The listing builds one solid part. Answer for the finished solid, in the listing's coordinates (mm). Face numbers are marked on the shaded views. Give positions to 0.01 mm unless a question says otherwise; leave off trailing zeros. Order: outer loops, then holes, each group sorted by start corner. A loop starts at its lowest first (then second) coordinate and runs counter-clockwise, first axis right, second up. Notation, with made-up numbers: (-8.75, -35) - (13.25, -35) arc R30 ccw to (13.25, -8) - close; hole circle Ø9 at (15, 28). An arc over 180 degrees is marked (long way). Answer in a Markdown table with one row per item. Add a question column.
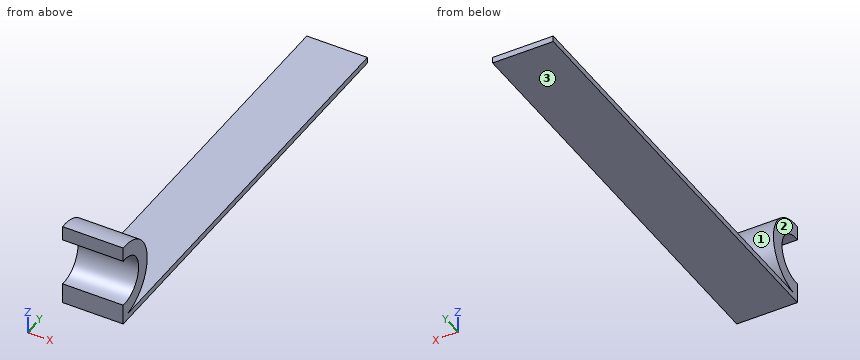
```python
from build123d import *

# Parameters (mm, degrees)
F0_W     = 25.4
F0_H     = 177.8
F1_DEPTH = 2.54
F4_DEPTH = 25.4


with BuildPart() as f1:
    # F0 (on Top) → F1 (new body)
    with BuildSketch(Plane.XY):
        with Locations((-51.181969, 33.563137)):
            Rectangle(F0_W, F0_H)
    extrude(amount=F1_DEPTH)

    # F3 (on face) → F4 (join)
    with BuildSketch(Plane.YZ.offset(-63.881969)):
        with BuildLine():
            Line((-55.336863, 8.636), (-55.336863, 2.54))
            ThreePointArc((-55.336863, 2.54), (-37.867352, 18.739499), (-55.336863, 34.938998))
            Line((-55.336863, 34.938998), (-55.336863, 28.842998))
            ThreePointArc((-55.336863, 28.842998), (-44.106861, 18.739499), (-55.336863, 8.636))
        make_face()
    extrude(amount=F4_DEPTH)


solid = f1.part
```
(1) The mould has two halves that part along Z. Classify the marked faces 1, 2 and 3: +Z half, -Z half, draft (parallel to the pull), parting line (faces both ways), or undercut.
(2) Each of these flat-tipped pins is pushed along its axis until it touches: P1, Ø6, axis at x = -52, z = 13.5, coming from the +Y side; P2, Ø3, axis at x = -52, y = 74, coming from the +Z side; P3, Ø1.5, axis at x = -43.5, z = 5, coming from the +Y side. Where does it stop, or does it pass through?
(3) Find section B-B, the plane y = 23. Write down the section's boundary in (x, z), plus the area to 3 significant figures.
(4) Find section C-C, the plane z = 26. Write down the section's boundary in (x, y), plus the area to 3 significant figures.
(5) Straight lines are drawn through the part: line 1 (Z direction, x = -60.75, y = 58); line 2 (Y direction, x = -50.5, z = 19); line 3 (Y direction, x = -54.75, z = 16). For each, find the intervals that lie inside material, in ascending order.
Answer key:
| question | item | result |
|---|---|---|
| 1 | face 1 | undercut |
| 1 | face 2 | draft |
| 1 | face 3 | -Z half |
| 2 | P1 | y = -38.02 |
| 2 | P2 | z = 2.54 |
| 2 | P3 | y = -44.36 |
| 3 | outline | (-63.88, 0) - (-38.48, 0) - (-38.48, 2.54) - (-63.88, 2.54) - close |
| 3 | area | 64.5 mm² |
| 4 | outline | (-63.88, -47.16) - (-38.48, -47.16) - (-38.48, -39.58) - (-63.88, -39.58) - close |
| 4 | area | 193 mm² |
| 5 | line 1 | 0 to 2.54 |
| 5 | line 2 | -44.11 to -37.87 |
| 5 | line 3 | -44.48 to -38.1 |
